```python
from build123d import *

# Parameters (mm, degrees)
SKETCH_1_R          = 22.5
EXTRUDE_1_DEPTH     = 4
SKETCH_2_R          = 17.5
EXTRUDE_2_DEPTH     = 15
SKETCH_3_R          = 1.5
SKETCH_3_W          = 20
SKETCH_3_H          = 20
CUT_EXTRUDE_1_DEPTH = 38.06076092


with BuildPart() as part:
    # 草图1 → 凸台-拉伸1 (new body)
    with BuildSketch(Plane.XY):
        Circle(SKETCH_1_R)
    extrude(amount=EXTRUDE_1_DEPTH)

    # 草图2 → 凸台-拉伸2 (add)
    with BuildSketch(Plane(origin=(0, 0, 0), x_dir=(-1, 0, 0), z_dir=(0, 0, -1))):
        Circle(SKETCH_2_R)
    extrude(amount=EXTRUDE_2_DEPTH)

    # 草图3 → 切除-拉伸1 (cut, through all)
    with BuildSketch(Plane.XY.offset(4)):
        with BuildLine():
            ThreePointArc((-8.5, -10), (-8.939339828, -8.939339828), (-10, -8.5))
            Line((-10, -8.5), (-10, -10))
            Line((-10, -10), (-8.5, -10))
        make_face()
        with BuildLine():
            Line((-10, -10), (-10, -8.5))
            ThreePointArc((-10, -8.5), (-11.060660172, -11.060660172), (-8.5, -10))
            Line((-8.5, -10), (-10, -10))
        make_face()
        with Locations((-10, -10)):
            Circle(SKETCH_3_R)
        with Locations((10, -10)):
            Circle(SKETCH_3_R)
        with Locations((10, 10)):
            Circle(SKETCH_3_R)
        with Locations((-10, 10)):
            Circle(SKETCH_3_R)
        Rectangle(SKETCH_3_W, SKETCH_3_H)
        with BuildLine():
            ThreePointArc((11.5, -10), (11.060660172, -8.939339828), (10, -8.5))
            Line((10, -8.5), (10, -10))
            Line((10, -10), (8.5, -10))
            ThreePointArc((8.5, -10), (10, -11.5), (11.5, -10))
        make_face()
        with BuildLine():
            Line((10, -10), (10, -8.5))
            ThreePointArc((10, -8.5), (8.939339828, -8.939339828), (8.5, -10))
            Line((8.5, -10), (10, -10))
        make_face()
        with BuildLine():
            ThreePointArc((11.5, 10), (10, 11.5), (8.5, 10))
            Line((8.5, 10), (10, 10))
            Line((10, 10), (10, 8.5))
            ThreePointArc((10, 8.5), (11.060660172, 8.939339828), (11.5, 10))
        make_face()
        with BuildLine():
            Line((10, 10), (8.5, 10))
            ThreePointArc((8.5, 10), (8.939339828, 8.939339828), (10, 8.5))
            Line((10, 8.5), (10, 10))
        make_face()
        with BuildLine():
            Line((-10, 8.5), (-10, 10))
            Line((-10, 10), (-8.5, 10))
            ThreePointArc((-8.5, 10), (-11.060660172, 11.060660172), (-10, 8.5))
        make_face()
        with BuildLine():
            Line((-8.5, 10), (-10, 10))
            Line((-10, 10), (-10, 8.5))
            ThreePointArc((-10, 8.5), (-8.939339828, 8.939339828), (-8.5, 10))
        make_face()
    extrude(amount=-CUT_EXTRUDE_1_DEPTH, mode=Mode.SUBTRACT)


solid = part.part
```
Geometry: final body of the model. Coordinates: model frame, mm. A direction names the side the tool comes from. Round coordinates to 2 decimals unless told otherwise and drop trailing zeros. Write each loop counter-clockwise with the first axis right and the second up, starting at its lowest first coordinate (ties: lowest second). Pieces come first, ordered by that corner, then holes. Notation, with made-up numbers: (85, -27.75) -> (140, -27.75) arc R6 ccw to (140, -20.75) -> close; hole circle Ø2 at (56, 86.25). An arc over 180 degrees is marked (long way). Return JSON: item names as keys, results as strings.
Q1. Section C-C on z = -5.25. Return the cut outline in (x, y), and give its area (3 significant figures).
From the geometry:
{"outline": "circle Ø35 at (0, 0); hole (-10, -8.5) arc R1.5 ccw (long way) to (-8.5, -10) -> (8.5, -10) arc R1.5 ccw (long way) to (10, -8.5) -> (10, 8.5) arc R1.5 ccw (long way) to (8.5, 10) -> (-8.5, 10) arc R1.5 ccw (long way) to (-10, 8.5) -> close", "area": "541 mm2"}
Q2. Set-up query: faces 4 (the flat face through (-10, 0, -5)), 5 (the flat face through (0, -11, -15)). Return all of +Z, -Z, +X, -X, +Y, -Y with unobstructed straight access to the full face (end or side cutting, diameter ignored); none if empty.
From the geometry:
{"face 4": "+Z, -Z", "face 5": "-Z, +X, -X, +Y, -Y"}
Q3. Section D-D on y = -14. Return the cut outline in (x, z).
From the geometry:
{"outline": "(-17.61, 0) -> (-10.5, 0) -> (-10.5, -15) -> (10.5, -15) -> (10.5, 0) -> (17.61, 0) -> (17.61, 4) -> (-17.61, 4) -> close"}
Q4. Mould query, pull axis Y, two halves, no side actions, for faces 1 (the flat face through (10, 0, -5)), 2 (the flat face through (12, -13, 0)), 3 (the cylindrical face through (13.887, -10.648, -7.395)). Classes: +Y half, -Y half, draft (parallel to the pull), parting line (faces both ways), or undercut.
From the geometry:
{"face 1": "undercut", "face 2": "draft", "face 3": "parting line"}
Q5. First-contact query: pin 1 Ø5 at (x, y) = (-10, 10) entering from -Z; pin 2 Ø3 at (x, z) = (14.5, -7.5) entering from -Y; pin 3 Ø6 at (x, z) = (10.5, 1.5) entering from -Y; pin 4 Ø4 at (x, z) = (-5, -5) entering from +Y. Flat tips, straight axial feed; report the tip coordinate or a pass-through.
From the geometry:
{"pin 1": "z = -15", "pin 2": "y = -11.72", "pin 3": "y = -21.21", "pin 4": "y = 17.24"}
Q6. Ray query, line 1 (X direction, y = 10.5, z = 2.25); line 2 (Z direction, x = 16, y = 13.5); line 3 (X direction, y = 2, z = -1). Return the intervals inside material, ascending.
From the geometry:
{"line 1": "-19.9 to -11.41, -8.59 to 8.59, 11.41 to 19.9", "line 2": "0 to 4", "line 3": "-17.39 to -10, 10 to 17.39"}
Q7. Section A-A on x = 0. Return the cut outline in (y, z), and give its area (3 significant figures).
From the geometry:
{"outline": "(-22.5, 0) -> (-17.5, 0) -> (-17.5, -15) -> (-10, -15) -> (-10, 4) -> (-22.5, 4) -> close; (10, -15) -> (17.5, -15) -> (17.5, 0) -> (22.5, 0) -> (22.5, 4) -> (10, 4) -> close", "area": "325 mm2"}
